Autodesk Inventor part; units mm, degrees
ref_plane "YZ Plane" through (0, 0, 0) normal (1, 0, 0) x (0, 1, 0)
ref_plane "XZ Plane" through (0, 0, 0) normal (0, 1, 0) x (-1, 0, 0)
ref_plane "XY Plane" through (0, 0, 0) normal (0, 0, 1) x (1, 0, 0)
sketch "Sketch1" plane through (0, 0, 0) normal (0, 0, 1) x (1, 0, 0)
  arc A0 (5.25, 0) -> (-5.25, 0) centre (0, 0) ccw
  arc A1 (10, 0) -> (-3.960396, 9.182334) centre (0, 0) ccw
  line L0 (-5.25, -8.511022) -> (-5.25, -20)
  line L1 (-5.25, -20) -> (-25.25, -20)
  line L2 (-25.25, -20) -> (-25.25, 0)
  line L3 (5.25, 0) -> (10, 0)
  line L4 (-25.25, 0) -> (-3.960396, 9.182334)
  line L5 (-5.25, -8.511022) -> (-5.25, 0)
  line L6 (-25.25, 0) -> (-25.25, 13)
  line L7 (-25.25, 13) -> (-10.25, 13)
  line L8 (-10.25, 13) -> (2.706976, 9.628622)
  point P0 (1.153738, 9.933221)
  point P1 (2.518133, 9.677758)
  dimension "d0" = 10.5
  dimension "d1" = 20
  dimension "d3" = 20
  dimension "d5" = 20
  dimension "d6" = 0
  dimension "d7" = 20
  dimension "d14" = 13
  dimension "d18" = 15
sketch "Sketch1 outline for Extrusion1" plane through (0, 0, 0) normal (0, 0, 1) x (1, 0, 0)
  arc A0 (10, 0) -> (2.518133, 9.677758) centre (0, 0) ccw
  line L0 (2.518133, 9.677758) -> (-10.25, 13)
  line L1 (-10.25, 13) -> (-25.25, 13)
  line L2 (-25.25, 13) -> (-25.25, -20)
  line L3 (-25.25, -20) -> (-5.25, -20)
  line L4 (-5.25, -20) -> (-5.25, 0)
  arc A1 (-5.25, 0) -> (5.25, 0) centre (0, 0) cw
  line L5 (5.25, 0) -> (10, 0)
extrude "Extrusion1" add sketch "Sketch1 outline for Extrusion1" along normal blind 17.5
sketch "Sketch3" plane through (0, 0, 17.5) normal (0, 0, 1) x (1, 0, 0)
  point P0 (0, 0)
sketch "Sketch4" plane through (0, 0, 0) normal (0, 0, -1) x (-1, 0, 0)
  arc A0 (-2.518133, 9.677758) -> (-10, 0) centre (0, 0) ccw
  line L0 (25.25, 13) -> (25.25, -20)
  arc A1 (-2.518133, 9.677758) -> (-10, 0) centre (0, 0) ccw
  line L1 (-5.25, 0) -> (-10, 0)
  arc A2 (5.25, 0) -> (-5.25, 0) centre (0, 0) ccw
  line L2 (5.25, -20) -> (5.25, 0)
  line L3 (25.25, -20) -> (5.25, -20)
  circle A3 centre (0, 0) radius 10
  line L4 (10, 11.228722) -> (10, -20)
  line L5 (25.25, -20) -> (5.25, -20)
  line L6 (10, 0) -> (25.25, 0)
  line L7 (25.25, 13) -> (25.25, -20)
  line L8 (10.25, 13) -> (25.25, 13)
  line L9 (-2.518133, 9.677758) -> (10.25, 13)
  point P0 (-1.153738, 9.933221)
extrude "Extrusion3" add sketch "Sketch4" along normal blind 10 contours L6 L0 L3 L4
fillet "Fillet1" radius 10 1 edges at (-17.625, 0, 0)
sketch "Sketch5" plane through (0, 0, 17.5) normal (0, 0, 1) x (1, 0, 0)
  line L0 (-25.25, 13) -> (-25.25, -20)
  line L1 (-25.25, -20) -> (-5.25, -20)
  line L2 (-5.25, -20) -> (-5.25, 0)
  arc A0 (5.25, 0) -> (-5.25, 0) centre (0, 0) ccw
  line L3 (5.25, 0) -> (10, 0)
  arc A1 (10, 0) -> (2.518133, 9.677758) centre (0, 0) ccw
  line L4 (2.518133, 9.677758) -> (-10.25, 13)
  line L5 (-10.25, 13) -> (-25.25, 13)
  circle A2 centre (-18.25, 8) radius 1.65
  circle A3 centre (-18.25, -2) radius 1.65
  dimension "d19" = 3.3
  dimension "d20" = 3.3
  dimension "d22" = 5
  dimension "d23" = 10
  dimension "d24" = 7
  dimension "d25" = 7
extrude "Extrusion4" cut sketch "Sketch5" against normal blind 15 contours A2 | A3
sketch "Sketch6" plane through (-25.25, -20, 17.5) normal (-1, 0, 0) x (0, 0, 1)
  line L0 (-7.5, 30.75) -> (-5, 30.75)
  line L1 (-5, 30.75) -> (-5, 25.25)
  line L2 (-5, 25.25) -> (-7.5, 25.25)
  line L3 (-7.5, 25.25) -> (-7.5, 30.75)
  line L4 (-7.5, 20.75) -> (-5, 20.75)
  line L5 (-5, 20.75) -> (-5, 15.25)
  line L6 (-5, 15.25) -> (-7.5, 15.25)
  line L7 (-7.5, 15.25) -> (-7.5, 20.75)
  line L8 (0, 19.65) -> (0, 16.35)
  line L9 (0, 29.65) -> (0, 26.35)
  point P0 (-17.5, 20)
  point P1 (-27.5, 16.35)
  point P2 (-27.5, 19.65)
  dimension "d28" = 5.5
  dimension "d29" = 5.5
  dimension "d30" = 2.5
  dimension "d31" = 2.5
  dimension "d32" = 0
  dimension "d33" = 5
  dimension "d34" = 3.3
  dimension "d35" = 1.1
  dimension "d36" = 1.1
  dimension "d37" = 1.1
  dimension "d38" = 1.1
extrude "Extrusion5" cut sketch "Sketch6" against normal blind 12
fillet "Fillet2" radius 3 1 edges at (-17.75, 13, 0)
equation "\"d7\" = d5"
equation "\"d29\" = d28"
equation "\"d31\" = d30"
equation "\"d35\" = -0.5 * d34 + 0.5 * d28"
equation "\"d37\" = d38"
properties part number "XAxisLimitSwitchMount"
The model under review builds one solid part; all positions refer to its coordinate system, in mm. A direction names the side the tool comes from. Round coordinates to 2 decimals unless told otherwise and drop trailing zeros. Write each loop counter-clockwise with the first axis right and the second up, starting at its lowest first coordinate (ties: lowest second). Pieces come first, ordered by that corner, then holes. Notation, with made-up numbers: (20, -30.75) - (72, -30.75) arc R27 cw to (72, 0.25) - close; hole circle Ø7 at (10, 18). An arc over 180 degrees is marked (long way). One line per question, with ' | ' between items.
Item 1: For P1, Ø2, axis at x = 2.5, z = 9.5, coming from the -Y side; P2, Ø1, axis at x = 4.5, z = 11.5, coming from the +Y side; P3, Ø0.8, axis at y = -1.5, z = 11, coming from the -X side, all flat-tipped, find the tip position at first contact; note any pin that passes through.
Resolved:
P1: stops at y = 3.91 | P2: stops at y = 9.17 | P3: stops at x = -13.25
Item 2: Add section D-D, the plane x = 0. Give the boundary of the cut face in (y, z).
Resolved:
outline: (5.25, 0) - (10, 0) arc R3 ccw to (10.33, 0.02) - (10.33, 17.5) - (5.25, 17.5) - close
Item 3: The part is to be moulded in two halves that separate along X. For faces 1 (the face through (-25.25, -3, 4)), 2 (the face through (-19.466, 9.115, 15.035)), 3 (the face through (-19.56, -3, 6.3)), 4 (the face through (-12, -3, 17.5)), say which applies: pulls with the +X half, pulls with the -X half, needs draft (parallel to the pull), parting line crosses it, or undercut.
Resolved:
face 1: pulls with the -X half | face 2: undercut | face 3: undercut | face 4: needs draft
Item 4: Add section C-C, the plane z = 11. Give the boundary of the cut face in (x, y).
Resolved:
outline: (-25.25, -20) - (-5.25, -20) - (-5.25, 0) arc R5.25 cw to (5.25, 0) - (10, 0) arc R10 ccw to (2.52, 9.68) - (-10.25, 13) - (-25.25, 13) - (-25.25, 10.75) - (-13.25, 10.75) - (-13.25, 5.25) - (-25.25, 5.25) - (-25.25, 0.75) - (-13.25, 0.75) - (-13.25, -4.75) - (-25.25, -4.75) - close
Item 5: Add section A-A, the plane y = -2. Give the boundary of the cut face in (x, z), then the cut area to 3 significant figures.
Resolved:
outline: (-25.25, -10) - (-10, -10) - (-10, 0) - (-5.25, 0) - (-5.25, 17.5) - (-16.6, 17.5) - (-16.6, 12.5) - (-13.25, 12.5) - (-13.25, 10) - (-16.6, 10) - (-16.6, 2.5) - (-19.9, 2.5) - (-19.9, 10) - (-25.25, 10) - close; (-25.25, 12.5) - (-19.9, 12.5) - (-19.9, 17.5) - (-25.25, 17.5) - close | area: 431 mm2
Item 6: Add section B-B, the plane z = 15. Give the boundary of the cut face in (x, y).
Resolved:
outline: (-25.25, -20) - (-5.25, -20) - (-5.25, 0) arc R5.25 cw to (5.25, 0) - (10, 0) arc R10 ccw to (2.52, 9.68) - (-10.25, 13) - (-25.25, 13) - close; hole circle Ø3.3 at (-18.25, -2); hole circle Ø3.3 at (-18.25, 8)
Item 7: For faces 5 (the face through (-19, 0.75, 11)), 6 (the face through (-18, -2, 2.5)), 7 (the face through (8, 0, 9)), list the 3-axis set-ups (+Z, -Z, +X, -X, +Y, -Y) from which the entire face can be reached by the end or side of a thin tool; tool diameter is ignored.
Resolved:
face 5: -X | face 6: +Z | face 7: +Z, -Z, +X, -Y
Item 8: To check wall thickness, follow probe 1 along Y at (x, z) = (-18.25, 14.8); probe 2 along Y at (x, z) = (-19.5, 8); probe 3 along Z at (x, y) = (-15.5, -3.5). State the ranges of each line that lie inside material, in increasing order.
Resolved:
probe 1: y = -20 to -3.65, -0.35 to 6.35, 9.65 to 13 | probe 2: y = -20 to -3.08, -0.92 to 6.92, 9.08 to 13 | probe 3: z = -10 to 10, 12.5 to 17.5
